```python
from build123d import *

# Parameters (mm, degrees)
F0_W     = 50.8
F0_H     = 50.8
F1_DEPTH = 50.8
F3_R     = 5.08
F4_T     = -2.54


# Not quite as in the source:
# - a shell that OpenCascade refuses in one call is made with other operations: the cavity is built on its own and cut out


with BuildPart() as f1:
    # F0 (on Top) → F1 (new body)
    with BuildSketch(Plane.XY):
        with Locations((-29.015717721, -32.2184429228)):
            Rectangle(F0_W, F0_H)
    extrude(amount=F1_DEPTH)

    # F3
    f3_edges = [f1.edges().sort_by_distance(p)[0] for p in [
        (-29.015718, -57.618443, 50.8),
        (-54.415718, -32.218443, 50.8),
        (-29.015718, -6.818443, 50.8),
        (-3.615718, -32.218443, 50.8),
        (-54.415718, -57.618443, 25.4),
        (-54.415718, -6.818443, 25.4),
        (-3.615718, -6.818443, 25.4),
        (-3.615718, -57.618443, 25.4),
        (-3.615718, -32.218443, 0),
    ]]
    fillet(f3_edges, radius=F3_R)

    # F4: a shell. OpenCascade refuses it in one call, so the cavity is built on its own and cut out:
    # the body offset inwards by the wall thickness, plus a prism from it out through each open face.
    f4_core = offset(f1.part, amount=F4_T, mode=Mode.PRIVATE)
    f4_exits = [f4_core.faces().sort_by_distance(p)[0] for p in [
        (-6.155718, -32.218443, 25.4),
    ]]
    add(f4_core, mode=Mode.SUBTRACT)
    extrude(f4_exits, amount=-F4_T, mode=Mode.SUBTRACT)


solid = f1.part
```
Work out the finished part from the listing and answer in its coordinate system (mm). A direction names the side the tool comes from. Round coordinates to 2 decimals unless told otherwise and drop trailing zeros. Write each loop counter-clockwise with the first axis right and the second up, starting at its lowest first coordinate (ties: lowest second). Pieces come first, ordered by that corner, then holes.
1) Flat-ended cylindrical pins translate along their axes: P1, Ø3, axis at y = -34.5, z = 34.5, coming from the +X side; P2, Ø8, axis at x = -33.5, y = -15.5, coming from the -Z side; P3, Ø2, axis at x = -4.5, y = -32, coming from the -Z side; P4, Ø2, axis at x = -4.5, z = 15.5, coming from the +Y side. Find the tip coordinate at first contact, or state that the pin passes through.
2) A cutting plane is placed at A-A on z = 38. Determine the outline of the cut face in (x, y), and give its area (3 significant figures).
3) Consider probe 1 along Y at (x, z) = (-29.5, 46); probe 2 along Z at (x, y) = (-32.5, -14); probe 3 along X at (y, z) = (-49, 37.5). Determine where each line is inside the solid, lowest interval first.
4) Which of the six approach directions +Z, -Z, +X, -X, +Y, -Y give full straight-line access (tool end or side, diameter ignored) to faces 4 (the face through (-51.151, -54.315, 24.432)), 5 (the face through (-5.06, -8.35, 23.18))?
5) A cutting plane is placed at C-C on y = -23. Determine the outline of the cut face in (x, z), and give its area (3 significant figures).
6) Determine the mould class of faces 1 (the face through (-5.06, -31.93, 49.27)), 2 (the face through (-54.416, -33, 23)), 3 (the face through (-51.15, -10.12, 24.43)) for opening direction X: pulls with the +X half, pulls with the -X half, needs draft (parallel to the pull), parting line crosses it, or undercut.
7) A cutting plane is placed at B-B on x = -32.5. Determine the outline of the cut face in (y, z).
Entries:
1. P1: stops at x = -51.88
1. P2: stops at z = 0
1. P3: stops at z = 1.13
1. P4: stops at y = -7.95
2. outline: (-54.42, -52.54) arc R5.08 ccw to (-49.34, -57.62) - (-8.7, -57.62) arc R5.08 ccw to (-3.62, -52.54) - (-6.16, -52.54) arc R2.54 cw to (-8.7, -55.08) - (-49.34, -55.08) arc R2.54 cw to (-51.88, -52.54) - (-51.88, -11.9) arc R2.54 cw to (-49.34, -9.36) - (-8.7, -9.36) arc R2.54 cw to (-6.16, -11.9) - (-3.62, -11.9) arc R5.08 ccw to (-8.7, -6.82) - (-49.34, -6.82) arc R5.08 ccw to (-54.42, -11.9) - close
2. area: 370 mm2
3. probe 1: y = -57.61 to -55.06, -9.37 to -6.83
3. probe 2: z = 0 to 2.54, 48.26 to 50.8
3. probe 3: x = -54.42 to -51.88
4. face 4: none
4. face 5: +Z, -Z, +X, +Y
5. outline: (-54.42, 0) - (-8.7, 0) arc R5.08 ccw to (-3.62, 5.08) - (-6.16, 5.08) arc R2.54 cw to (-8.7, 2.54) - (-51.88, 2.54) - (-51.88, 45.72) arc R2.54 cw to (-49.34, 48.26) - (-8.7, 48.26) arc R2.54 cw to (-6.16, 45.72) - (-3.62, 45.72) arc R5.08 ccw to (-8.7, 50.8) - (-49.34, 50.8) arc R5.08 ccw to (-54.42, 45.72) - close
5. area: 375 mm2
6. face 1: pulls with the +X half
6. face 2: pulls with the -X half
6. face 3: undercut
7. outline: (-57.62, 0) - (-6.82, 0) - (-6.82, 45.72) arc R5.08 ccw to (-11.9, 50.8) - (-52.54, 50.8) arc R5.08 ccw to (-57.62, 45.72) - close; hole (-55.08, 2.54) - (-9.36, 2.54) - (-9.36, 45.72) arc R2.54 ccw to (-11.9, 48.26) - (-52.54, 48.26) arc R2.54 ccw to (-55.08, 45.72) - close
